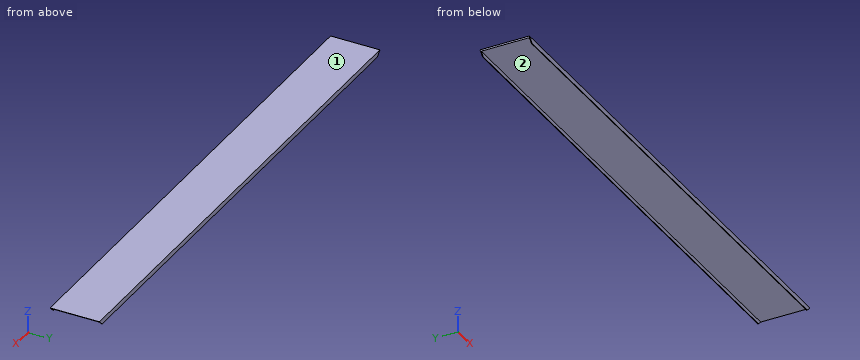
```python
from build123d import *

# Parameters (mm, degrees)
CROQUIS1_W              = 1056
CROQUIS1_H              = 10
SALIENTE_EXTRUIR1_DEPTH = 100
CORTAR_EXTRUIR1_DEPTH   = 100
CROQUIS3_W              = 1056
CROQUIS3_H              = 97.5
CORTAR_EXTRUIR2_DEPTH   = 8


with BuildPart() as part:
    # Croquis1 → Saliente-Extruir1 (new body)
    with BuildSketch(Plane(origin=(0, 0, 0), x_dir=(1, 0, 0), z_dir=(0, 1, 0))):
        Rectangle(CROQUIS1_W, CROQUIS1_H)
    extrude(amount=SALIENTE_EXTRUIR1_DEPTH)

    # Croquis2 → Cortar-Extruir1 (cut)
    with BuildSketch(Plane(origin=(0, 100, 0), x_dir=(1, 0, 0), z_dir=(0, 1, 0))):
        Polygon((-528, -5), (-518, 5), (-528, 5), align=None)
        Polygon((518, 5), (528, 5), (528, -5), align=None)
    extrude(amount=-CORTAR_EXTRUIR1_DEPTH, mode=Mode.SUBTRACT)

    # Croquis3 → Cortar-Extruir2 (cut)
    with BuildSketch(Plane(origin=(0, 0, -5), x_dir=(-1, 0, 0), z_dir=(0, 0, -1))):
        with Locations((0, 50)):
            Rectangle(CROQUIS3_W, CROQUIS3_H)
    extrude(amount=-CORTAR_EXTRUIR2_DEPTH, mode=Mode.SUBTRACT)


solid = part.part
```
The model under review builds one solid part; all positions refer to its coordinate system, in mm. Face numbers are marked on the shaded views. A direction names the side the tool comes from. Round coordinates to 2 decimals unless told otherwise and drop trailing zeros. Write each loop counter-clockwise with the first axis right and the second up, starting at its lowest first coordinate (ties: lowest second). Pieces come first, ordered by that corner, then holes. Notation, with made-up numbers: M 50,30.5 L 92,30.5 A18 cw 92,43.5 Z; hole C -30,-15 d10. An arc over 180 degrees is marked long. Use CSV: the item, a comma, the result in double quotes. Start each with the question number.
(1) We need section C-C, the plane y = 62.5. State the section outline as (x, z) points, then the cut area to 3 significant figures.
(2) We need section A-A, the plane z = -3.25. State the section outline as (x, y) points, then the cut area to 3 significant figures.
(3) Tool access review of the marked faces 1 and 2: name each direction out of +Z, -Z, +X, -X, +Y, -Y from which nothing blocks a thin tool from reaching the whole face with its end or side.
(4) We need section B-B, the plane x = 68. State the section outline as (y, z) points.
(5) Clearance check with flat-ended pins moving along their axes: P1, Ø12, axis at x = 264.5, y = 16.5, coming from the -Z side; P2, Ø2, axis at y = 47, z = 2.5, coming from the -X side. State where each tip first meets the part, or that it passes through.
(6) For line 1 along Y through (x, z) = (336, -0.75); line 2 along Z through (x, y) = (69.5, 54); line 3 along X through (y, z) = (55, 3.5), list the stretches that pass through material, from the lowest coordinate up.
Findings:
1,outline,"M -528,5 L -526,3 L 526,3 L 528,5 Z"
1,area,"2,110 mm^2"
2,outline,"M -519.75,0 L 519.75,0 L 519.75,1.25 L -519.75,1.25 Z; M -519.75,98.75 L 519.75,98.75 L 519.75,100 L -519.75,100 Z"
2,area,"2,600 mm^2"
3,face 1,"+Z, +X, -X, +Y, -Y"
3,face 2,"-Z, +X, -X"
4,outline,"M 0,-5 L 1.25,-5 L 1.25,3 L 98.75,3 L 98.75,-5 L 100,-5 L 100,5 L 0,5 Z"
5,P1,"z = 3"
5,P2,"x = -526.5"
6,line 1,"0 to 1.25, 98.75 to 100"
6,line 2,"3 to 5"
6,line 3,"-526.5 to 526.5"
